from build123d import *

# Parameters (mm, degrees)
SKETCH1_R           = 1.5
SKETCH1_R_2         = 1.866773139
BOSS_EXTRUDE2_DEPTH = 3


with BuildPart() as part:
    # Sketch1 → Boss-Extrude2 (new body)
    with BuildSketch(Plane.XY):
        with BuildLine():
            Line((19.955328479, -21.686654411), (19.955328479, -7.686654411))
            Line((19.955328479, -7.686654411), (15.62520146, -5.186654411))
            Line((15.62520146, -5.186654411), (15.42520146, -4.686654411))
            Line((15.42520146, -4.686654411), (15.62520146, -4.186654411))
            Line((15.62520146, -4.186654411), (15.42520146, -3.686654411))
            Line((15.42520146, -3.686654411), (15.62520146, -3.186654411))
            Line((15.62520146, -3.186654411), (15.42520146, -2.686654411))
            Line((15.42520146, -2.686654411), (15.62520146, -2.186654411))
            Line((15.62520146, -2.186654411), (15.42520146, -1.686654411))
            Line((15.42520146, -1.686654411), (15.62520146, -1.186654411))
            Line((15.62520146, -1.186654411), (15.42520146, -0.686654411))
            Line((15.42520146, -0.686654411), (15.62520146, -0.186654411))
            Line((15.62520146, -0.186654411), (15.42520146, 0.313345589))
            Line((15.42520146, 0.313345589), (15.62520146, 0.813345589))
            Line((15.62520146, 0.813345589), (15.42520146, 1.313345589))
            Line((15.42520146, 1.313345589), (15.62520146, 1.813345589))
            Line((15.62520146, 1.813345589), (15.42520146, 2.313345589))
            Line((15.42520146, 2.313345589), (15.62520146, 2.813345589))
            Line((15.62520146, 2.813345589), (15.42520146, 3.313345589))
            Line((15.42520146, 3.313345589), (15.42520146, 3.802153535))
            ThreePointArc((15.42520146, 3.802153535), (21.487107687, 3.455011814), (25.455328479, -1.140685983))
            Line((25.455328479, -1.140685983), (25.455328479, -21.140685983))
            ThreePointArc((25.455328479, -21.140685983), (25.995551768, -26.504062064), (27.594518651, -31.651969317))
            Line((27.594518651, -31.651969317), (35.020472422, -49.140685983))
            ThreePointArc((35.020472422, -49.140685983), (32.372376923, -55.697178203), (25.815884703, -53.049082704))
            Line((25.815884703, -53.049082704), (16.435732572, -30.958072179))
            ThreePointArc((16.435732572, -30.958072179), (16.267997475, -26.710838203), (18.95611766, -23.418249345))
            ThreePointArc((18.95611766, -23.418249345), (19.687607088, -22.686259743), (19.955328479, -21.686654411))
        make_face()
        with Locations((30.418178563, -51.094884343)):
            Circle(SKETCH1_R, mode=Mode.SUBTRACT)
        with Locations((19.62520146, -2.186654411)):
            Circle(SKETCH1_R_2, mode=Mode.SUBTRACT)
        with Locations((21.958485203, -28.613034147)):
            Circle(SKETCH1_R, mode=Mode.SUBTRACT)
    extrude(amount=BOSS_EXTRUDE2_DEPTH)


solid = part.part
The model under review builds one solid part; all positions refer to its coordinate system, in mm. A direction names the side the tool comes from. Coordinates: 2 decimals unless noted, no trailing zeros. Write each loop counter-clockwise with the first axis right and the second up, starting at its lowest first coordinate (ties: lowest second). Pieces come first, ordered by that corner, then holes. Notation, with made-up numbers: (-34, 15.25) - (-16, 15.25) arc R26 ccw to (-16, 29.25) - close; hole circle Ø7 at (54, -8.5). An arc over 180 degrees is marked (long way). Answer as a JSON object with one key per item and string values. Group by question number.
1. Add section D-D (x = 34.25). Give the boundary of the cut face in (y, z), plus the area to 3 significant figures.
2. To check wall thickness, follow probe 1 along Y at (x, z) = (19.5, 0.3); probe 2 along Y at (x, z) = (23, 1.65); probe 3 along X at (y, z) = (-11, 0.4). State the ranges of each line that lie inside material, in increasing order.
3. Add section A-A (x = 30.25). Give the boundary of the cut face in (y, z).
4. Add section C-C (y = -17.5). Give the boundary of the cut face in (x, z).
5. Machinability: for faces 5 (the face through (21.191, -42.158, 1.479)), 6 (the face through (19.68, -22.7, 1.48)), 7 (the face through (25.455, -11, 1)), which of the approach directions +Z, -Z, +X, -X, +Y, -Y give a long, thin tool a straight path to every point of the face, cutting with its end or side? Answer none if there is none.
6. Clearance check with flat-ended pins moving along their axes: pin 1 Ø1 at (x, y) = (18, -39) entering from -Z; pin 2 Ø1 at (y, z) = (-22.5, 1.5) entering from +X; pin 3 Ø0.9 at (y, z) = (-13, 1.5) entering from -X. State where each tip first meets the part, or that it passes through.
7. Mouldability with a two-part tool opening along X and no side actions: class faces 1 (the face through (31.849, -50.644, 1.479)), 2 (the face through (17.76, -2.1, 1.48)), 3 (the face through (31.256, -40.274, 1.479)), 4 (the face through (16.25, -26.77, 1.48)) as pulls with the +X half, pulls with the -X half, needs draft (parallel to the pull), parting line crosses it, or undercut.
8. Add section B-B (z = 2.4). Give the number of separate pieces and of enclosed holes in the cut face, plus the area to 3 significant figures.
Findings:
{
 "1": {"outline": "(-54.31, 0) - (-47.33, 0) - (-47.33, 3) - (-54.31, 3) - close", "area": "20.9 mm²"},
 "2": {"probe 1": "-38.17 to -22.96, -7.42 to -4.05, -0.32 to 4.12", "probe 2": "-46.42 to -29.69, -27.53 to 2.48", "probe 3": "19.96 to 25.46"},
 "3": {"outline": "(-56.09, 0) - (-52.59, 0) - (-52.59, 3) - (-56.09, 3) - close; (-49.6, 0) - (-37.91, 0) - (-37.91, 3) - (-49.6, 3) - close"},
 "4": {"outline": "(19.96, 0) - (25.46, 0) - (25.46, 3) - (19.96, 3) - close"},
 "5": {"face 5": "+Z, -Z, -X, -Y", "face 6": "+Z, -Z, -X", "face 7": "+Z, -Z, +X, +Y"},
 "6": {"pin 1": "through", "pin 2": "x = 25.52", "pin 3": "x = 19.96"},
 "7": {"face 1": "undercut", "face 2": "undercut", "face 3": "pulls with the +X half", "face 4": "pulls with the -X half"},
 "8": {"separate pieces": "1", "enclosed holes": "3", "area": "495 mm²"}
}
